Verification items for the finished model (mm, model axes). Face numbers are marked on the shaded views. A direction names the side the tool comes from. Round coordinates to 2 decimals unless told otherwise and drop trailing zeros. Order: outer loops, then holes, each group sorted by start corner. A loop starts at its lowest first (then second) coordinate and runs counter-clockwise, first axis right, second up. Notation, with made-up numbers: (45, 64.25) -> (89, 64.25) arc R21 cw to (89, 91.25) -> close; hole circle Ø5 at (-34, 75). An arc over 180 degrees is marked (long way). Return JSON: item names as keys, results as strings. Group by question number.
Item 1: Scan lines: probe 1 along Y at (x, z) = (-1, 8) (3 decimals); probe 2 along Y at (x, z) = (3.75, 1.5) (3 decimals); probe 3 along X at (y, z) = (2.25, 9). Record each from-to range of solid material in increasing order. Write a range as from..to.
Item 2: Sectioned sample at D-D on z = 6.5. Record the cut outline in (x, y) (3 decimals).
Item 3: Access from +Z, -Z, +X, -X, +Y, -Y to the whole of each face (thin tool, end or side, straight path). Record for the marked faces 5, 6 and 7.
Item 4: Draft check along Y on the marked faces 1, 2, 3 and 4. Enter one of: pulls with the +Y half, pulls with the -Y half, needs draft (parallel to the pull), parting line crosses it, or undercut.
Item 5: Sectioned sample at B-B on x = 2.25. Record the cut outline in (y, z) (3 decimals), plus the area to 3 significant figures.
Item 6: Depth check by flat-ended pin: pin 1 Ø3 at (y, z) = (-2, 8) entering from +X; pin 2 Ø1.6 at (x, y) = (-4.5, -4.5) entering from +Z; pin 3 Ø1.5 at (y, z) = (-1.5, 5) entering from -X. Enter the tip coordinate at first touch or a pass-through.
Item 7: Sectioned sample at A-A on z = 8.75. Record the cut outline in (x, y) (3 decimals), plus the area to 3 significant figures.
Item 8: Sectioned sample at C-C on x = -5.75. Record the cut outline in (y, z) (3 decimals), plus the area to 3 significant figures.
```python
from build123d import *

# Parameters (mm, degrees)
CROQUIS1_W              = 7.32
CROQUIS1_H              = 11.65
SALIENTE_EXTRUIR1_DEPTH = 3.52
CROQUIS2_W              = 7.32
CROQUIS2_H              = 4.2
CROQUIS2_H_2            = 4.01
SALIENTE_EXTRUIR2_DEPTH = 6.16
CROQUIS3_R              = 1.29
SALIENTE_EXTRUIR3_DEPTH = 2.05


with BuildPart() as part:
    # Croquis1 → Saliente-Extruir1 (new body)
    with BuildSketch(Plane.XY):
        Rectangle(CROQUIS1_W, CROQUIS1_H)
    extrude(amount=SALIENTE_EXTRUIR1_DEPTH)

    # Croquis2 → Saliente-Extruir2 (add)
    with BuildSketch(Plane.XY.offset(3.52)):
        with Locations((0, -3.725)):
            Rectangle(CROQUIS2_W, CROQUIS2_H)
        with Locations((0, 3.82)):
            Rectangle(CROQUIS2_W, CROQUIS2_H_2)
    extrude(amount=SALIENTE_EXTRUIR2_DEPTH)

    # Croquis3 → Saliente-Extruir3 (add)
    # profile 1 of 2: a face of its own
    with BuildSketch(Plane(origin=(0, -5.825, 0), x_dir=(-1, 0, 0), z_dir=(0, -1, 0))):
        with BuildLine():
            ThreePointArc((-6.0536211, -1.27), (-9.0586211, -4.275), (-6.0536211, -7.28))
            Line((-6.0536211, -7.28), (-3.66, -7.28))
            Line((-3.66, -7.28), (-3.66, -1.27))
            Line((-3.66, -1.27), (-6.0536211, -1.27))
        make_face()
        with Locations(Location((-6.0536211, -4.275, 0), (0, 0, 90))):
            Circle(CROQUIS3_R, mode=Mode.SUBTRACT)
    # profile 2 of 2: a face of its own
    with BuildSketch(Plane(origin=(0, -5.825, 0), x_dir=(-1, 0, 0), z_dir=(0, -1, 0))):
        with BuildLine():
            ThreePointArc((6.0536211, -7.28), (9.0586211, -4.275), (6.0536211, -1.27))
            Line((6.0536211, -1.27), (3.66, -1.27))
            Line((3.66, -1.27), (3.66, -7.28))
            Line((3.66, -7.28), (6.0536211, -7.28))
        make_face()
        with Locations(Location((6.0536211, -4.275, 0), (0, 0, 90))):
            Circle(CROQUIS3_R, mode=Mode.SUBTRACT)
    extrude(amount=-SALIENTE_EXTRUIR3_DEPTH)


solid = part.part
```
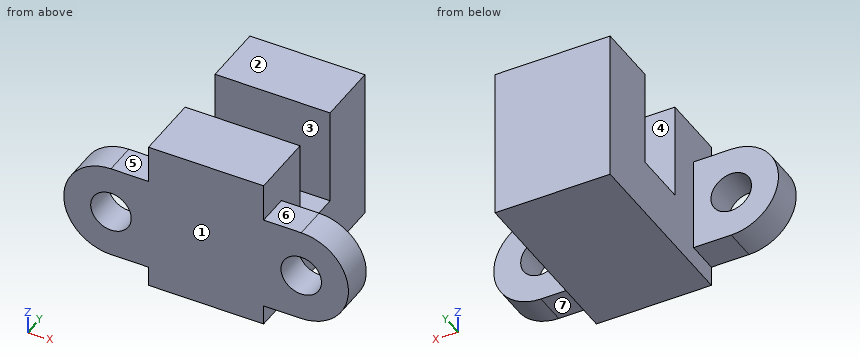
Recorded:
{
 "1": {"probe 1": "-5.825..-1.625, 1.815..5.825", "probe 2": "-5.825..-3.775", "probe 3": "-3.66..3.66"},
 "2": {"outline": "(-8.073, -5.825) -> (8.073, -5.825) -> (8.073, -3.775) -> (3.66, -3.775) -> (3.66, -1.625) -> (-3.66, -1.625) -> (-3.66, -3.775) -> (-8.073, -3.775) -> close; (-3.66, 1.815) -> (3.66, 1.815) -> (3.66, 5.825) -> (-3.66, 5.825) -> close"},
 "3": {"face 5": "+Z, -X, +Y, -Y", "face 6": "+Z, +X, +Y, -Y", "face 7": "-Z, +X, +Y, -Y"},
 "4": {"face 1": "pulls with the -Y half", "face 2": "needs draft", "face 3": "undercut", "face 4": "undercut"},
 "5": {"outline": "(-5.825, 0) -> (5.825, 0) -> (5.825, 9.68) -> (1.815, 9.68) -> (1.815, 3.52) -> (-1.625, 3.52) -> (-1.625, 9.68) -> (-5.825, 9.68) -> close", "area": "91.6 mm²"},
 "6": {"pin 1": "x = 3.66", "pin 2": "z = 7.28", "pin 3": "x = -3.66"},
 "7": {"outline": "(-3.66, -5.825) -> (3.66, -5.825) -> (3.66, -1.625) -> (-3.66, -1.625) -> close; (-3.66, 1.815) -> (3.66, 1.815) -> (3.66, 5.825) -> (-3.66, 5.825) -> close", "area": "60.1 mm²"},
 "8": {"outline": "(-5.825, 1.27) -> (-3.775, 1.27) -> (-3.775, 3.021) -> (-5.825, 3.021) -> close; (-5.825, 5.529) -> (-3.775, 5.529) -> (-3.775, 7.28) -> (-5.825, 7.28) -> close", "area": "7.18 mm²"}
}
